```python
from build123d import *

# Parameters (mm, degrees)
F0_R     = 11.1183318615
F1_DEPTH = 25.4
F2_DEPTH = 12.7
F3_DEPTH = 12.7
F4_DEPTH = 12.7762
F5_DEPTH = 0.508
F6_DEPTH = 11.938


with BuildPart() as f1:
    # F0 (on Top) → F1 (new body)
    with BuildSketch(Plane.XY):
        Polygon((-47.498, 63.5), (-63.5, 63.5), (-63.5, 0), (-47.498, 0), (-47.498, 7.874), (-16.002, 7.874), (-16.002, 0), (0, 0), (0, 63.5), (-16.002, 63.5), (-16.002, 55.626), (-47.498, 55.626), align=None)
        with Locations((-31.75, 31.75)):
            Circle(F0_R, mode=Mode.SUBTRACT)
    extrude(amount=F1_DEPTH)

    # F2 (add): a face of the model
    f2_faces = [f1.faces().sort_by_distance(p)[0] for p in [
        (-55.499, 62.6019743879, 25.4),
    ]]
    extrude(f2_faces, amount=F2_DEPTH)

    # F3 (cut): a face of the model
    f3_faces = [f1.faces().sort_by_distance(p)[0] for p in [
        (-55.499, 62.6019743879, 38.1),
    ]]
    extrude(f3_faces, amount=-F3_DEPTH, mode=Mode.SUBTRACT)

    # F4 (cut): a face of the model
    f4_faces = [f1.faces().sort_by_distance(p)[0] for p in [
        (-55.499, 62.6019743879, 25.4),
    ]]
    extrude(f4_faces, amount=-F4_DEPTH, mode=Mode.SUBTRACT)

    # F0 (on Top) → F5 (join)
    with BuildSketch(Plane.XY):
        with Locations((-31.75, 31.75)):
            Circle(F0_R)
    extrude(amount=F5_DEPTH)

    # F6 (add): a face of the model
    f6_faces = [f1.faces().sort_by_distance(p)[0] for p in [
        (-31.75, 31.75, 0.508),
    ]]
    extrude(f6_faces, amount=F6_DEPTH)


solid = f1.part
```
The listing builds one solid part. Answer for the finished solid, in the listing's coordinates (mm). A direction names the side the tool comes from. Coordinates: 2 decimals unless noted, no trailing zeros. Write each loop counter-clockwise with the first axis right and the second up, starting at its lowest first coordinate (ties: lowest second). Pieces come first, ordered by that corner, then holes. Notation, with made-up numbers: (78.5, 85) -> (115.5, 85) arc R25 ccw to (115.5, 107) -> close; hole circle Ø7 at (5.25, -15). An arc over 180 degrees is marked (long way). Write each question's results on one line, items separated by ' | '. Start each with the question number.
1) A cutting plane is placed at B-B (x = -31.75). Determine the outline of the cut face in (y, z).
2) Flat-ended cylindrical pins translate along their axes: pin 1 Ø1 at (x, y) = (-38.5, 24) entering from +Z; pin 2 Ø5 at (x, z) = (-22, 9.5) entering from +Y. Find the tip coordinate at first contact, or state that the pin passes through.
3) A cutting plane is placed at D-D (x = -40.5). Determine the outline of the cut face in (y, z), then the cut area to 3 significant figures.
4) Straight lines are drawn through the part: probe 1 along X at (y, z) = (58, 8.5); probe 2 along Y at (x, z) = (-31.5, 6.5); probe 3 along Z at (x, y) = (-24, 30). For each, find the intervals that lie inside material, in ascending order.
5) A cutting plane is placed at A-A (y = 58). Determine the outline of the cut face in (x, z).
6) A tool of negligible diameter and unlimited length cuts with its end or side. For faces 5 (the flat face through (-32, 32, 0)), 6 (the flat face through (-32, 55.626, 6)), 7 (the flat face through (-16.002, 4, 6)), 8 (the flat face through (-32, 32, 12.446)), from which of +Z, -Z, +X, -X, +Y, -Y can it reach the whole face along a straight path? Write none if from no direction.
7) For a pull along X with two mould halves and no side action, classify faces 1 (the flat face through (-63.5, 32, 6)), 2 (the flat face through (-56, 0, 6)), 3 (the flat face through (-16.002, 60, 6)), 4 (the flat face through (0, 31, 6)) as +X half, -X half, draft (parallel to the pull), parting line (faces both ways), or undercut.
8) A cutting plane is placed at C-C (z = 10.25). Determine the outline of the cut face in (x, y).
Values follow:
1) outline: (7.87, 0) -> (55.63, 0) -> (55.63, 12.62) -> (42.87, 12.62) -> (42.87, 12.45) -> (20.63, 12.45) -> (20.63, 12.62) -> (7.87, 12.62) -> close
2) pin 1: z = 12.45 | pin 2: y = 55.63
3) outline: (7.87, 0) -> (55.63, 0) -> (55.63, 12.62) -> (38.61, 12.62) -> (38.61, 12.45) -> (24.89, 12.45) -> (24.89, 12.62) -> (7.87, 12.62) -> close | area: 600 mm²
4) probe 1: -63.5 to -47.5, -16 to 0 | probe 2: 7.87 to 55.63 | probe 3: 0 to 12.45
5) outline: (-63.5, 0) -> (-47.5, 0) -> (-47.5, 12.62) -> (-63.5, 12.62) -> close; (-16, 0) -> (0, 0) -> (0, 12.62) -> (-16, 12.62) -> close
6) face 5: -Z, +X, -X, +Y, -Y | face 6: +Z, -Z, +Y | face 7: +Z, -Z, -Y | face 8: +Z
7) face 1: -X half | face 2: draft | face 3: undercut | face 4: +X half
8) outline: (-63.5, 0) -> (-47.5, 0) -> (-47.5, 7.87) -> (-16, 7.87) -> (-16, 0) -> (0, 0) -> (0, 63.5) -> (-16, 63.5) -> (-16, 55.63) -> (-47.5, 55.63) -> (-47.5, 63.5) -> (-63.5, 63.5) -> close
